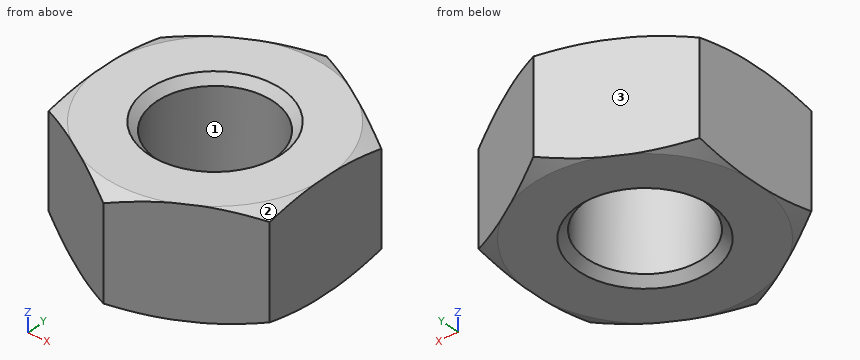
```python
from build123d import *

# Parameters (mm, degrees)
SKETCH_1_R      = 2.1
EXTRUDE_1_DEPTH = 3.89


with BuildPart() as part:
    # 스케치1 → 보스-돌출1 (new body)
    with BuildSketch(Plane.XY):
        Polygon((0, 4.618802154), (-4, 2.309401077), (-4, -2.309401077), (0, -4.618802154), (4, -2.309401077), (4, 2.309401077), align=None)
        Circle(SKETCH_1_R, mode=Mode.SUBTRACT)
    extrude(amount=EXTRUDE_1_DEPTH)

    # 스케치3 → 컷-회전3 (revolve, cut)
    with BuildSketch(Plane(origin=(0, 0, 0), x_dir=(1, 0, 0), z_dir=(0, 1, 0)), mode=Mode.PRIVATE) as cut_revolve_3_sk:
        Polygon((2.09, 0.001), (2.09, -0.299), (2.39, 0.001), align=None)
        Polygon((4, 0.01), (4.65, 0.01), (4.65, -0.29), align=None)
        Polygon((4.65, -3.6), (4, -3.9), (4.65, -3.9), align=None)
        Polygon((2.39, -3.891), (2.09, -3.891), (2.09, -3.591), align=None)
    revolve(cut_revolve_3_sk.sketch.rotate(Axis((0, 0, 1.945), (0, 0, -1)), 180), axis=Axis((0, 0, 1.945), (0, 0, -1)), mode=Mode.SUBTRACT)


solid = part.part
```
Read the model definition and answer for the solid it produces. Units are mm, in the model's axes. Face numbers are marked on the shaded views. Coordinates: 2 decimals unless noted, no trailing zeros. Loops run counter-clockwise (first coordinate to the right, second up) from the corner with the lowest first, then second, coordinate; pieces in that order, holes last.
(1) Consider line 1 along X through (y, z) = (0, 1.6); line 2 along X through (y, z) = (1, 0.35); line 3 along Y through (x, z) = (-1, 3.75). Determine where each line is inside the solid, lowest interval first.
Solution:
line 1: x = -4 to -2.1, 2.1 to 4
line 2: x = -4 to -1.85, 1.85 to 4
line 3: y = -4.04 to -2.01, 2.01 to 4.04
(2) The part is cut by section B-B (z = 3.3). Determine the outline of the cut face in (x, y), and give its area (3 significant figures).
Solution:
outline: (-4, -2.31) - (0, -4.62) - (4, -2.31) - (4, 2.31) - (0, 4.62) - (-4, 2.31) - close; hole circle Ø4.2 at (0, 0)
area: 41.6 mm2
(3) The mould has two halves that part along X. Classify the marked faces 1, 2 and 3: released by +X, released by -X, zero draft, split by the parting line, or undercut.
Solution:
face 1: undercut
face 2: released by +X
face 3: released by -X
(4) The part is cut by section A-A (y = 0). Determine the outline of the cut face in (x, z).
Solution:
outline: (-4, 0) - (-2.39, 0) - (-2.1, 0.29) - (-2.1, 3.6) - (-2.39, 3.89) - (-4, 3.89) - close; (2.1, 0.29) - (2.39, 0) - (4, 0) - (4, 3.89) - (2.39, 3.89) - (2.1, 3.6) - close
(5) Flat-ended cylindrical pins translate along their axes: pin 1 Ø1.5 at (x, z) = (1.5, 2) entering from +Y; pin 2 Ø1 at (x, z) = (-2, 0.5) entering from +Y; pin 3 Ø4 at (x, y) = (0, 0) entering from -Z. Find the tip coordinate at first contact, or state that the pin passes through.
Solution:
pin 1: stops at y = 4.19
pin 2: stops at y = 3.75
pin 3: passes through
